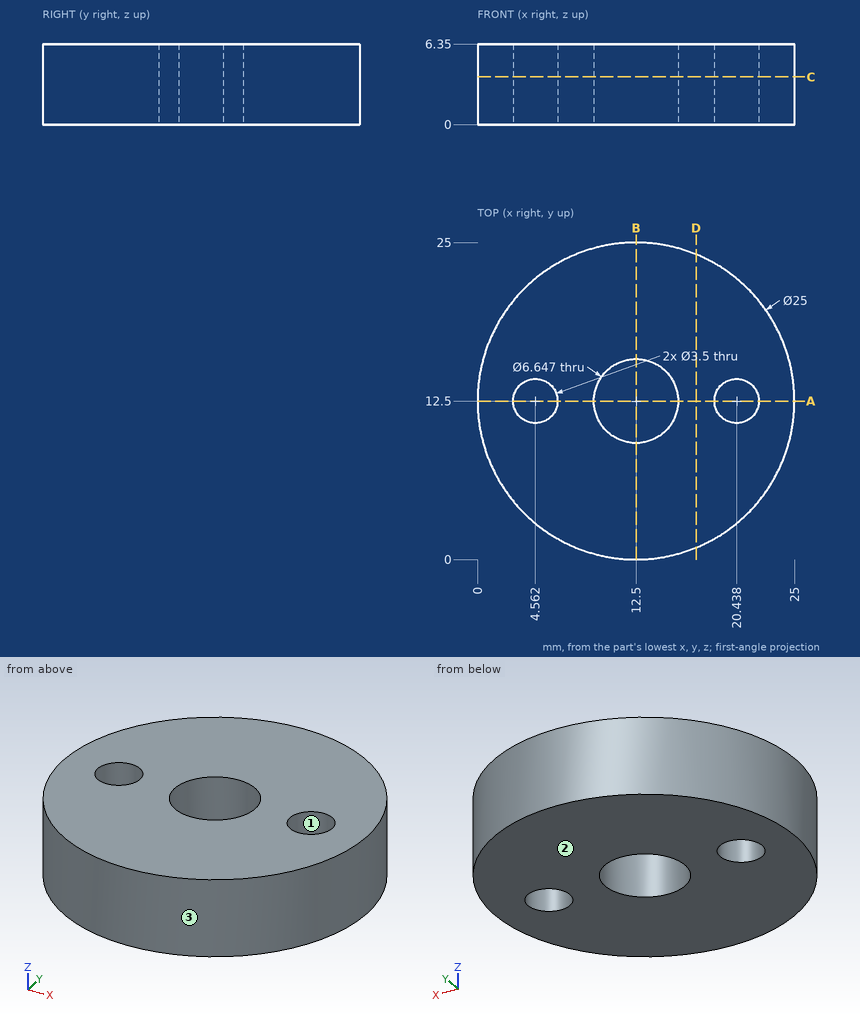
For this review, use the dimensioned drawing (mm, ordinates from the lowest corner) and the shaded views. Round coordinates to 2 decimals unless told otherwise and drop trailing zeros. Order: outer loops, then holes, each group sorted by start corner. A loop starts at its lowest first (then second) coordinate and runs counter-clockwise, first axis right, second up. Notation, with made-up numbers: (14.5, -22) - (31.5, -22) arc R16 ccw to (31.5, -4) - close; hole circle Ø1 at (73.5, -25.75). An arc over 180 degrees is marked (long way). Use one line per item in the form item = value.
Q1. Mouldability with a two-part tool opening along Y and no side actions: class the marked faces 1, 2 and 3 as pulls with the +Y half, pulls with the -Y half, needs draft (parallel to the pull), parting line crosses it, or undercut.
Response values:
face_1 = undercut
face_2 = needs draft
face_3 = parting line crosses it
Q2. Add section B-B on x = 12.5. Give the boundary of the cut face in (y, z).
Response values:
outline = (0, 0) - (9.18, 0) - (9.18, 6.35) - (0, 6.35) - close; (15.82, 0) - (25, 0) - (25, 6.35) - (15.82, 6.35) - close
Q3. Add section A-A on y = 12.5. Give the boundary of the cut face in (x, z).
Response values:
outline = (0, 0) - (2.81, 0) - (2.81, 6.35) - (0, 6.35) - close; (6.31, 0) - (9.18, 0) - (9.18, 6.35) - (6.31, 6.35) - close; (15.82, 0) - (18.69, 0) - (18.69, 6.35) - (15.82, 6.35) - close; (22.19, 0) - (25, 0) - (25, 6.35) - (22.19, 6.35) - close
Q4. Add section D-D on x = 17.25. Give the boundary of the cut face in (y, z).
Response values:
outline = (0.94, 0) - (24.06, 0) - (24.06, 6.35) - (0.94, 6.35) - close
Q5. Add section C-C on z = 3.75. Give the boundary of the cut face in (x, y).
Response values:
outline = circle Ø25 at (12.5, 12.5); hole circle Ø3.5 at (4.56, 12.5); hole circle Ø6.65 at (12.5, 12.5); hole circle Ø3.5 at (20.44, 12.5)
Q6. Clearance check with flat-ended pins moving along their axes: P1, Ø5.5, axis at x = 12.5, y = 12.5, coming from the +Z side; P2, Ø1, axis at y = 20.5, z = 2, coming from the +X side. State where each tip first meets the part, or that it passes through.
Response values:
P1 = through
P2 = 22.5
Q7. To check wall thickness, follow line 1 (X direction, y = 13.5, z = 4.5) (1 decimal); line 2 (Y direction, x = 19.25, z = 4.5) (1 decimal); line 3 (Y direction, x = 20.75, z = 1.75). State the ranges of each line that lie inside material, in increasing order.
Response values:
line_1 = 0 to 3.1, 6 to 9.3, 15.7 to 19, 21.9 to 25
line_2 = 2 to 11.2, 13.8 to 23
line_3 = 3.11 to 10.78, 14.22 to 21.89
